Check sheet for the modelled part. Datum: model origin and axes. Units: mm. Face numbers are marked on the shaded views. A direction names the side the tool comes from. Give positions to 0.01 mm unless a question says otherwise; leave off trailing zeros. Order: outer loops, then holes, each group sorted by start corner. A loop starts at its lowest first (then second) coordinate and runs counter-clockwise, first axis right, second up. Notation, with made-up numbers: (57, -18) -> (104, -18) arc R5 cw to (104, -11) -> close; hole circle Ø6 at (-15.75, 5.25). An arc over 180 degrees is marked (long way). Answer in a Markdown table with one row per item. Add a question column.
(1) Cross-section at A-A (y = 38.5). Record the cut outline in (x, z), then the cut area to 3 significant figures.
(2) Cross-section at D-D (x = 7). Record the cut outline in (y, z), then the cut area to 3 significant figures.
(3) Go/stop test with flat-tipped pins: pin 1 (3 mm diameter, centred on y = 23.5, z = 7.5, fed in from -X); pin 2 (1.5 mm diameter, centred on x = 6, z = 0.5, fed in from +Y); pin 3 (8 mm diameter, centred on x = 9, z = -7, fed in from -Y); pin 4 (5.5 mm diameter, centred on x = -24, z = 2, fed in from +Y). Record where each tip stops, or that it passes through.
(4) Set-up check for the marked faces 1, 2, 3, 4 and 5: record each of +Z, -Z, +X, -X, +Y, -Y from which the full face is reachable in a straight line by a thin tool's end or side.
(5) Cross-section at C-C (z = 4.75). Record the cut outline in (x, y), then the cut area to 3 significant figures.
(6) Thickness scan on L1, parallel to Y at x = 3.5, z = 7.25; L2, parallel to X at y = 32.5, z = 9; L3, parallel to Y at x = 24, z = -3.25. Record the ranges inside material, lowest first. Write a range as [from, to].
(7) Cross-section at B-B (x = -8). Record the cut outline in (y, z).
```python
from build123d import *

# Parameters (mm, degrees)
SKETCH1_W           = 40.26
SKETCH1_H           = 20
BOSS_EXTRUDE1_DEPTH = 36.86
SKETCH2_W           = 20
SKETCH2_H           = 2.6
BOSS_EXTRUDE2_DEPTH = 7.17
SKETCH3_W           = 20
SKETCH3_H           = 2.6
BOSS_EXTRUDE3_DEPTH = 7.17
SKETCH4_R           = 10
BOSS_EXTRUDE4_DEPTH = 2.48
SKETCH5_R           = 6.55
BOSS_EXTRUDE5_DEPTH = 1.56
SKETCH6_R           = 2.9
BOSS_EXTRUDE6_DEPTH = 4.2


with BuildPart() as part:
    # Sketch1 → Boss-Extrude1 (new body)
    with BuildSketch(Plane(origin=(0, 0, 0), x_dir=(1, 0, 0), z_dir=(0, 1, 0))):
        Rectangle(SKETCH1_W, SKETCH1_H)
    extrude(amount=BOSS_EXTRUDE1_DEPTH)

    # Sketch2 → Boss-Extrude2 (add)
    with BuildSketch(Plane(origin=(20.13, 0, 0), x_dir=(0, 0, -1), z_dir=(1, 0, 0))):
        with Locations((0, 29.3)):
            Rectangle(SKETCH2_W, SKETCH2_H)
    extrude(amount=BOSS_EXTRUDE2_DEPTH)

    # Sketch3 → Boss-Extrude3 (add)
    with BuildSketch(Plane.ZY.offset(20.13)):
        with Locations((0, 29.3)):
            Rectangle(SKETCH3_W, SKETCH3_H)
    extrude(amount=BOSS_EXTRUDE3_DEPTH)

    # Sketch4 → Boss-Extrude4 (add)
    with BuildSketch(Plane(origin=(0, 36.86, 0), x_dir=(1, 0, 0), z_dir=(0, 1, 0))):
        with Locations((-10.13, 0)):
            Circle(SKETCH4_R)
        with BuildLine():
            Line((13.87, 10), (-10.13, 10))
            ThreePointArc((-10.13, 10), (-3.058932188, 7.071067812), (-0.13, 0))
            ThreePointArc((-0.13, 0), (-3.058932188, -7.071067812), (-10.13, -10))
            Line((-10.13, -10), (13.87, -10))
            Line((13.87, -10), (13.87, 10))
        make_face()
    extrude(amount=BOSS_EXTRUDE4_DEPTH)

    # Sketch5 → Boss-Extrude5 (add)
    with BuildSketch(Plane(origin=(0, 39.34, 0), x_dir=(1, 0, 0), z_dir=(0, 1, 0))):
        with Locations((-10.13, 0)):
            Circle(SKETCH5_R)
    extrude(amount=BOSS_EXTRUDE5_DEPTH)

    # Sketch6 → Boss-Extrude6 (add)
    with BuildSketch(Plane(origin=(0, 40.9, 0), x_dir=(1, 0, 0), z_dir=(0, 1, 0))):
        with Locations((-10.13, 0)):
            Circle(SKETCH6_R)
    extrude(amount=BOSS_EXTRUDE6_DEPTH)


solid = part.part
```
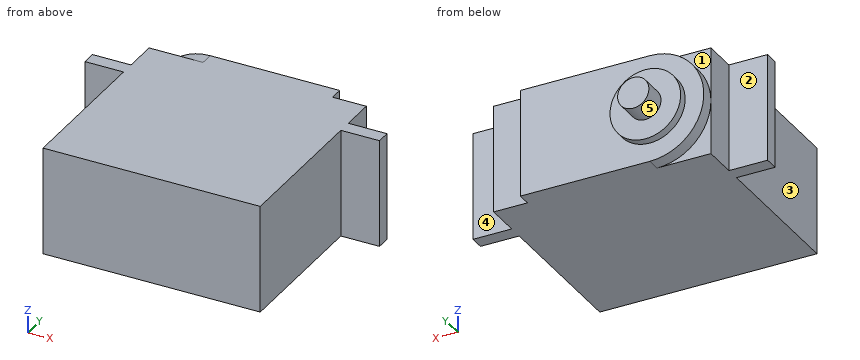
Answer below:
| question | item | result |
|---|---|---|
| 1 | outline | (-10.13, -10) -> (13.87, -10) -> (13.87, 10) -> (-10.13, 10) arc R10 ccw to start |
| 1 | area | 637 mm² |
| 2 | outline | (0, -10) -> (39.34, -10) -> (39.34, 10) -> (0, 10) -> close |
| 2 | area | 787 mm² |
| 3 | pin 1 | stops at x = -20.13 |
| 3 | pin 2 | stops at y = 39.34 |
| 3 | pin 3 | stops at y = 0 |
| 3 | pin 4 | stops at y = 30.6 |
| 4 | face 1 | +Z, -X, +Y |
| 4 | face 2 | +Z, -Z, -X, +Y |
| 4 | face 3 | +Z, -Z, -X, -Y |
| 4 | face 4 | +Z, -Z, +X, +Y |
| 4 | face 5 | +Y |
| 5 | outline | (-27.3, 28) -> (-20.13, 28) -> (-20.13, 0) -> (20.13, 0) -> (20.13, 28) -> (27.3, 28) -> (27.3, 30.6) -> (20.13, 30.6) -> (20.13, 36.86) -> (13.87, 36.86) -> (13.87, 39.34) -> (-5.62, 39.34) -> (-5.62, 40.9) -> (-14.64, 40.9) -> (-14.64, 39.34) -> (-18.93, 39.34) -> (-18.93, 36.86) -> (-20.13, 36.86) -> (-20.13, 30.6) -> (-27.3, 30.6) -> close |
| 5 | area | 1,620 mm² |
| 6 | L1 | y = [0, 39.34] |
| 6 | L2 | x = [-20.13, 20.13] |
| 6 | L3 | y = [28, 30.6] |
| 7 | outline | (0, -10) -> (39.34, -10) -> (39.34, -6.19) -> (40.9, -6.19) -> (40.9, -1.97) -> (45.1, -1.97) -> (45.1, 1.97) -> (40.9, 1.97) -> (40.9, 6.19) -> (39.34, 6.19) -> (39.34, 10) -> (0, 10) -> close |
